```python
from build123d import *

# Parameters (mm, degrees)
F1_W     = 228.6
F1_H     = 76.2
F2_DEPTH = 76.2
F3_W     = 76.2
F3_H     = 76.2
F4_DEPTH = 76.2


# Not quite as in the source:
# - a variable given as a bare number and used for a length is read in inches; the dataset says mm whatever the document's units were


with BuildPart() as f2:
    # F1 (on Front) → F2 (new body)
    with BuildSketch(Plane.XZ):
        Rectangle(F1_W, F1_H)
    extrude(amount=F2_DEPTH)

    # F3 (on face) → F4 (join)
    with BuildSketch(Plane.XZ.offset(76.2)):
        with Locations((-76.2, 0)):
            Rectangle(F3_W, F3_H)
    extrude(amount=F4_DEPTH)


solid = f2.part
```
The listing builds one solid part. Answer for the finished solid, in the listing's coordinates (mm). A direction names the side the tool comes from. Give positions to 0.01 mm unless a question says otherwise; leave off trailing zeros. Write each loop counter-clockwise with the first axis right and the second up, starting at its lowest first coordinate (ties: lowest second). Pieces come first, ordered by that corner, then holes. Notation, with made-up numbers: (89.25, -38) -> (118.25, -38) arc R21 cw to (118.25, -2) -> close; hole circle Ø8 at (28, 29). An arc over 180 degrees is marked (long way). Write item = value, one per line. Start each with the question number.
1) Which of the six approach directions +Z, -Z, +X, -X, +Y, -Y give full straight-line access (tool end or side, diameter ignored) to faces 1 (the face through (-2, 0, 1)), 2 (the face through (37, -76.2, 1))?
2) The part is cut by section A-A, the plane z = -30. Determine the outline of the cut face in (x, y).
3) Each of these flat-tipped pins is pushed along its axis until it touches: pin 1 (12 mm diameter, centred on y = -113.5, z = 2, fed in from +X); pin 2 (5 mm diameter, centred on x = 20, z = -28, fed in from -Y). Where does it stop, or does it pass through?
4) Straight lines are drawn through the part: line 1 along X through (y, z) = (-78, 29.5); line 2 along Y through (x, z) = (-18.5, -7.5). For each, find the intervals that lie inside material, in ascending order.
5) The part is cut by section C-C, the plane x = 81.5. Determine the outline of the cut face in (y, z).
6) The part is cut by section B-B, the plane y = -130.5. Determine the outline of the cut face in (x, z).
Solutions:
q1.face_1 = +Z, -Z, +X, -X, +Y
q1.face_2 = +Z, -Z, +X, -Y
q2.outline = (-114.3, -152.4) -> (-38.1, -152.4) -> (-38.1, -76.2) -> (114.3, -76.2) -> (114.3, 0) -> (-114.3, 0) -> close
q3.pin_1 = -38.1
q3.pin_2 = -76.2
q4.line_1 = -114.3 to -38.1
q4.line_2 = -76.2 to 0
q5.outline = (-76.2, -38.1) -> (0, -38.1) -> (0, 38.1) -> (-76.2, 38.1) -> close
q6.outline = (-114.3, -38.1) -> (-38.1, -38.1) -> (-38.1, 38.1) -> (-114.3, 38.1) -> close
